Job drawing, mm, ordinate dimensions from the low corner. One solid piece. A direction names the side the tool comes from. Give positions to 0.01 mm unless a question says otherwise; leave off trailing zeros. Write each loop counter-clockwise with the first axis right and the second up, starting at its lowest first coordinate (ties: lowest second). Pieces come first, ordered by that corner, then holes. Notation, with made-up numbers: (62.5, 18) - (100.5, 18) arc R18 ccw to (100.5, 36) - close; hole circle Ø4 at (55.25, 52). An arc over 180 degrees is marked (long way). Answer in a Markdown table with one row per item. Add a question column.
1. Which spindle directions (+Z, -Z, +X, -X, +Y, -Y) get a long thin tool onto all of the face, cutting with end or side? Do the marked faces 1 and 2. Say none if no direction does.
2. Band-saw the part on C-C on z = 5. Write the cut outline in (x, y).
3. Band-saw the part on D-D on x = 18.45. Write the cut outline in (y, z).
4. Band-saw the part on B-B on y = 4.5. Write the cut outline in (x, z).
5. Drop flat-ended pins along their axis: pin 1 Ø5.5 at (x, y) = (3, 3.5) entering from +Z; pin 2 Ø3.5 at (x, y) = (3.45, 23.45) entering from +Z. Give the stop position or say it passes through.
6. Band-saw the part on A-A on x = 3.45. Write the cut outline in (y, z).
7. Probe line 1 along Y through (x, z) = (3.45, 2.35); line 2 along Y through (x, z) = (3.45, 1); line 3 along Y through (x, z) = (18.45, 6.35). List the from-to ranges inside material, lowest first.
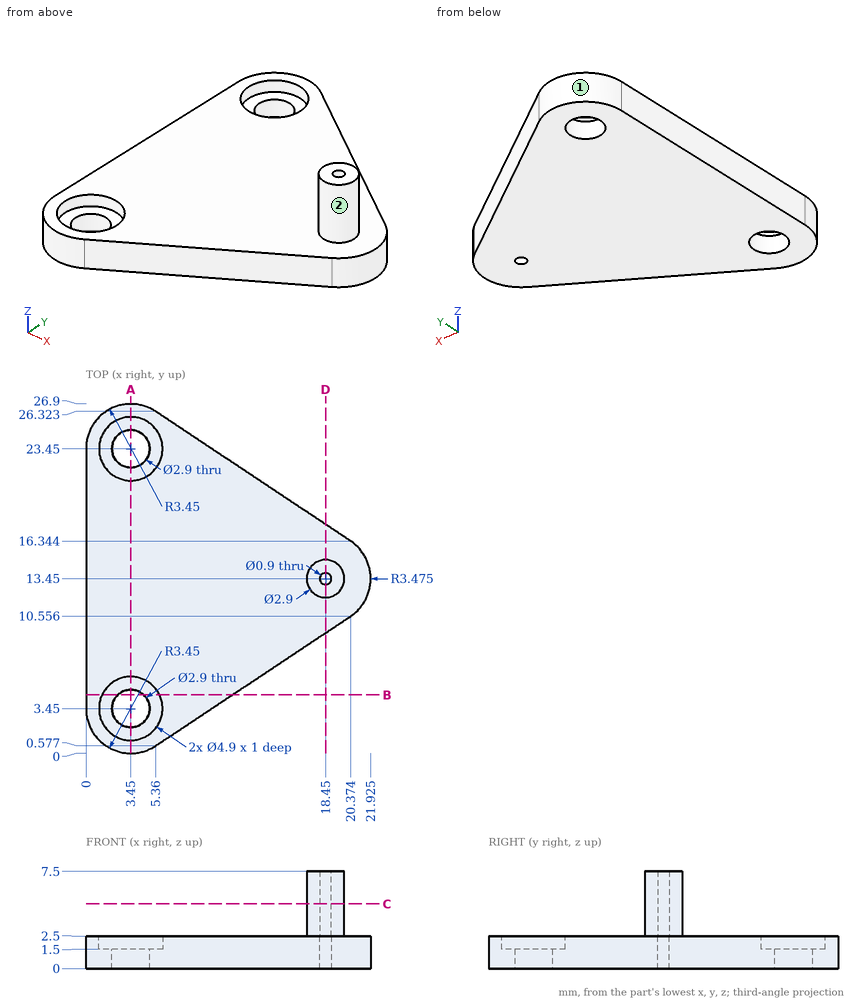
Values:
| question | item | result |
|---|---|---|
| 1 | face 1 | +Z, -Z, +Y |
| 1 | face 2 | +Z |
| 2 | outline | circle Ø2.9 at (18.45, 13.45); hole circle Ø0.9 at (18.45, 13.45) |
| 3 | outline | (9.28, 0) - (13, 0) - (13, 7.5) - (12, 7.5) - (12, 2.5) - (9.28, 2.5) - close; (13.9, 0) - (17.62, 0) - (17.62, 2.5) - (14.9, 2.5) - (14.9, 7.5) - (13.9, 7.5) - close |
| 4 | outline | (0, 0) - (2.45, 0) - (2.45, 1.5) - (1.24, 1.5) - (1.24, 2.5) - (0, 2.5) - close; (4.45, 0) - (11.26, 0) - (11.26, 2.5) - (5.66, 2.5) - (5.66, 1.5) - (4.45, 1.5) - close |
| 5 | pin 1 | stops at z = 2.5 |
| 5 | pin 2 | stops at z = 1.5 |
| 6 | outline | (0, 0) - (2, 0) - (2, 1.5) - (1, 1.5) - (1, 2.5) - (0, 2.5) - close; (4.9, 0) - (22, 0) - (22, 1.5) - (21, 1.5) - (21, 2.5) - (5.9, 2.5) - (5.9, 1.5) - (4.9, 1.5) - close; (24.9, 0) - (26.9, 0) - (26.9, 2.5) - (25.9, 2.5) - (25.9, 1.5) - (24.9, 1.5) - close |
| 7 | line 1 | y = 0 to 1, 5.9 to 21, 25.9 to 26.9 |
| 7 | line 2 | y = 0 to 2, 4.9 to 22, 24.9 to 26.9 |
| 7 | line 3 | y = 12 to 13, 13.9 to 14.9 |
